from build123d import *

# Parameters (mm, degrees)
SKETCH1_W           = 280
SKETCH1_H           = 236
BOSS_EXTRUDE1_DEPTH = 40
FILLET1_R           = 30
CUT_EXTRUDE2_DEPTH  = 8.25
FILLET2_R           = 2


with BuildPart() as part:
    # Sketch1 → Boss-Extrude1 (new body)
    with BuildSketch(Plane(origin=(0, 0, 0), x_dir=(1, 0, 0), z_dir=(0, 1, 0))):
        with Locations((27.44, -35.06)):
            Rectangle(SKETCH1_W, SKETCH1_H)
    extrude(amount=BOSS_EXTRUDE1_DEPTH)

    # Fillet1
    fillet1_edges = [part.edges().sort_by_distance(p)[0] for p in [
        (167.44, 40, 35.06),
        (27.44, 40, -82.94),
        (-112.56, 40, 35.06),
        (-112.56, 20, -82.94),
        (167.44, 20, -82.94),
        (167.44, 20, 153.06),
        (-112.56, 20, 153.06),
        (27.44, 40, 153.06),
    ]]
    fillet(fillet1_edges, radius=FILLET1_R)

    # Sketch3 → Cut-Extrude2 (cut)
    with BuildSketch(Plane(origin=(0, 40, 0), x_dir=(1, 0, 0), z_dir=(0, 1, 0))):
        with BuildLine():
            Line((-20.684825583, 17.14), (75.564825583, 17.14))
            ThreePointArc((75.564825583, 17.14), (83.172419453, 13.630340169), (85.44, 5.564903101))
            Line((85.44, 5.564903101), (79.315174417, -32.835096899))
            ThreePointArc((79.315174417, -32.835096899), (75.930340169, -38.86759387), (69.44, -41.26))
            Line((69.44, -41.26), (-14.56, -41.26))
            ThreePointArc((-14.56, -41.26), (-21.050340169, -38.86759387), (-24.435174417, -32.835096899))
            Line((-24.435174417, -32.835096899), (-30.56, 5.564903101))
            ThreePointArc((-30.56, 5.564903101), (-28.292419453, 13.630340169), (-20.684825583, 17.14))
        make_face()
    extrude(amount=-CUT_EXTRUDE2_DEPTH, mode=Mode.SUBTRACT)

    # Fillet2
    fillet2_edges = [part.edges().sort_by_distance(p)[0] for p in [
        (-21.050340169, 31.75, 38.86759387),
        (-27.497587208, 31.75, 13.635096899),
        (-28.292419453, 31.75, -13.630340169),
        (27.44, 31.75, -17.14),
        (83.172419453, 31.75, -13.630340169),
        (82.377587208, 31.75, 13.635096899),
        (75.930340169, 31.75, 38.86759387),
        (27.44, 31.75, 41.26),
    ]]
    fillet(fillet2_edges, radius=FILLET2_R)


solid = part.part
Source: CAD feature listing. Evaluate the final solid. Frame: model axes, mm. A direction names the side the tool comes from. Round coordinates to 2 decimals unless told otherwise and drop trailing zeros. Write each loop counter-clockwise with the first axis right and the second up, starting at its lowest first coordinate (ties: lowest second). Pieces come first, ordered by that corner, then holes. Notation, with made-up numbers: M -31,22 L -8,22 A25 cw -8,34 Z; hole C 83.25,58 d1. An arc over 180 degrees is marked long. One line per item, written item: value. Start each with the question number.
Item 1: Set-up query: faces 4 (the flat face through (-112.56, 5, 36)), 5 (the cylindrical face through (-20.975, 36.919, 38.931)). Return all of +Z, -Z, +X, -X, +Y, -Y with unobstructed straight access to the full face (end or side cutting, diameter ignored); none if empty.
Item 2: Pin query (flat end, axial travel): pin 1 (1.9 mm diameter, centred on x = 26.5, y = 37, fed in from -Z); pin 2 (6 mm diameter, centred on x = -61.5, y = 31.5, fed in from -Z); pin 3 (5 mm diameter, centred on x = -8, y = 15.5, fed in from +Z). Return the tip coordinate at first contact, or that it passes through.
Item 3: Ray query, L1, parallel to Z at x = 20, y = 37; L2, parallel to X at y = 11, z = 44.5; L3, parallel to Y at x = -19, z = -1. Return the intervals inside material, ascending. Write a range as from..to.
Item 4: Section query A-A (x = 28). Return the cut outline in (y, z), plus the area to 3 significant figures.
Item 5: Mould query, pull axis Z, two halves, no side actions, for faces 1 (the cylindrical face through (158.885, 5.07, -73.919)), 2 (the flat face through (26, 40, 53)), 3 (the flat face through (28, 37, 41.26)). Classes: pulls with the +Z half, pulls with the -Z half, needs draft (parallel to the pull), parting line crosses it, or undercut.
Item 6: Section query C-C (y = 21.5). Return the cut outline in (x, z).
Item 7: Section query D-D (x = 130). Return the cut outline in (y, z), plus the area to 3 significant figures.
Item 8: Section query B-B (z = 101). Return the cut outline in (x, y), plus the area to 3 significant figures.
Result set:
1. face 4: +Z, -Z, -X, +Y, -Y
1. face 5: +Y
2. pin 1: stops at z = -67.82
2. pin 2: stops at z = -76.56
2. pin 3: stops at z = 152.91
3. L1: z = -66.02..-17.14, 41.26..136.14
3. L2: x = -112.54..167.42
3. L3: y = 0..31.75
4. outline: M 0,-82.94 L 10,-82.94 A30 ccw 40,-52.94 L 40,-17.14 L 33.75,-17.14 A2 cw 31.75,-15.14 L 31.75,39.26 A2 cw 33.75,41.26 L 40,41.26 L 40,123.06 A30 ccw 10,153.06 L 0,153.06 Z
4. area: 8,570 mm²
5. face 1: pulls with the -Z half
5. face 2: needs draft
5. face 3: undercut
6. outline: M -110.27,-52.94 A27.71 ccw -82.56,-80.65 L 137.44,-80.65 A27.71 ccw 165.15,-52.94 L 165.15,123.06 A27.71 ccw 137.44,150.77 L -82.56,150.77 A27.71 ccw -110.27,123.06 Z
7. outline: M 0,-82.94 L 10,-82.94 A30 ccw 40,-52.94 L 40,123.06 A30 ccw 10,153.06 L 0,153.06 Z
7. area: 9,050 mm²
8. outline: M -112.56,0 L 167.44,0 L 167.44,10 A30 ccw 137.44,40 L -82.56,40 A30 ccw -112.56,10 Z
8. area: 10,800 mm²
